Here's the drawing with two shaded views (mm, measured from the low corner). I have some questions. A direction names the side the tool comes from. Round coordinates to 2 decimals unless told otherwise and drop trailing zeros. Order: outer loops, then holes, each group sorted by start corner. A loop starts at its lowest first (then second) coordinate and runs counter-clockwise, first axis right, second up. Notation, with made-up numbers: M 55.25,45 L 66.25,45 A25 ccw 66.25,77 Z; hole C -15,13.25 d2. An arc over 180 degrees is marked long. One line per question, with ' | ' between items.
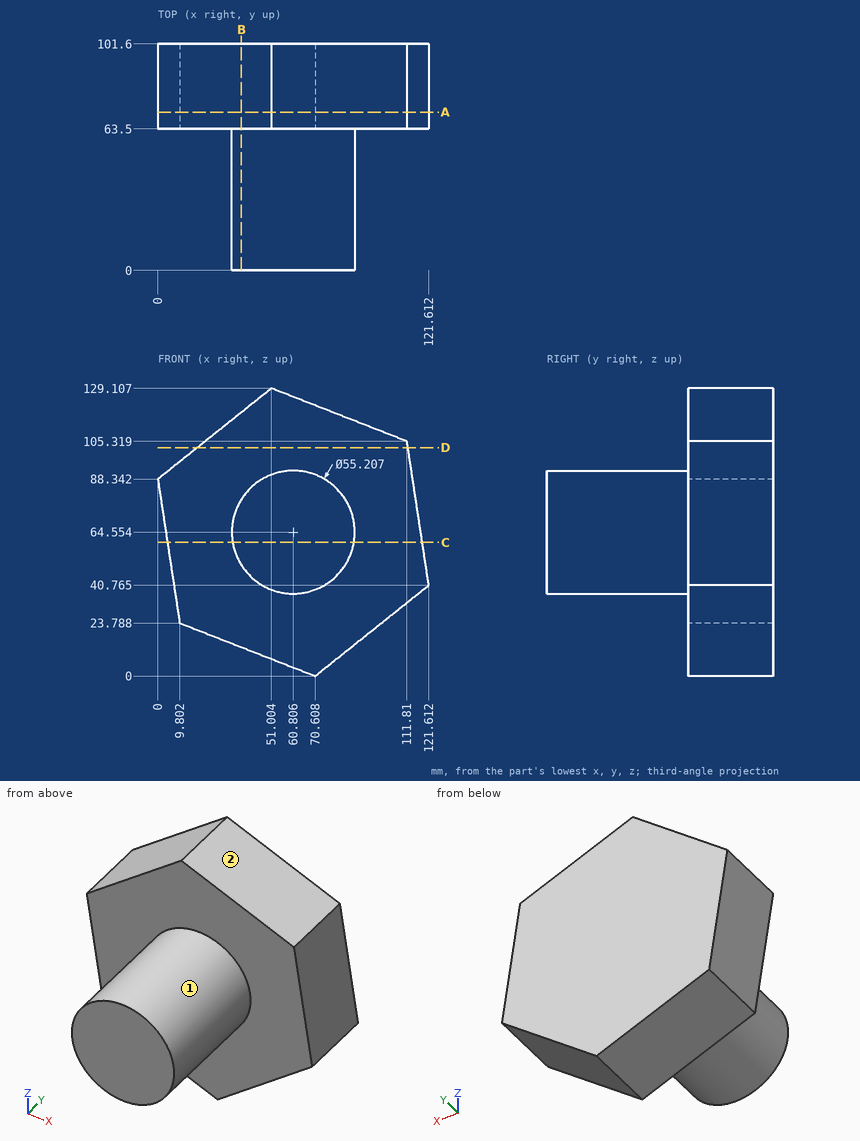
(1) On a 3-axis mill with a long thin cutter (end or side, diameter ignored), from which of +Z, -Z, +X, -X, +Y, -Y can I reach the whole of each face in a straight line? I mean the marked faces 1 and 2. Say none if no direction works.
Final values:
face 1: -Y | face 2: +Z, +X, +Y, -Y
(2) If we section it at B-B on x = 37.5: Please give me the cut outline in (y, z) (1 decimal).
Final values:
outline: M 0,49.8 L 63.5,49.8 L 63.5,13 L 101.6,13 L 101.6,118.3 L 63.5,118.3 L 63.5,79.3 L 0,79.3 Z
(3) Will this pin go through, and if not, where does the flat tip stop? pin 1 Ø12 at (x, z) = (30.5, 103) entering from -Y.
Final values:
pin 1: y = 63.5
(4) If we section it at A-A on y = 71: Please give me the cut outline in (x, z) (1 decimal), plus the area to 3 significant figures.
Final values:
outline: M 0,88.3 L 9.8,23.8 L 70.6,0 L 121.6,40.8 L 111.8,105.3 L 51,129.1 Z | area: 11,100 mm^2
(5) If we section it at C-C on z = 60: Please give me the cut outline in (x, y).
Final values:
outline: M 4.3,63.5 L 33.58,63.5 L 33.58,0 L 88.03,0 L 88.03,63.5 L 118.69,63.5 L 118.69,101.6 L 4.3,101.6 Z
(6) If we section it at D-D on z = 102.5: Please give me the cut outline in (x, y), plus the area to 3 significant figures.
Final values:
outline: M 17.71,63.5 L 112.24,63.5 L 112.24,101.6 L 17.71,101.6 Z | area: 3,600 mm^2
(7) Please list where these lines run through material, in increasing order: probe 1 along Y at (x, z) = (88, 38); probe 2 along Z at (x, y) = (60, 42) (1 decimal); probe 3 along Z at (x, y) = (56.5, 21). Write a range as [from, to].
Final values:
probe 1: [63.5, 101.6] | probe 2: [37, 92.1] | probe 3: [37.29, 91.82]
